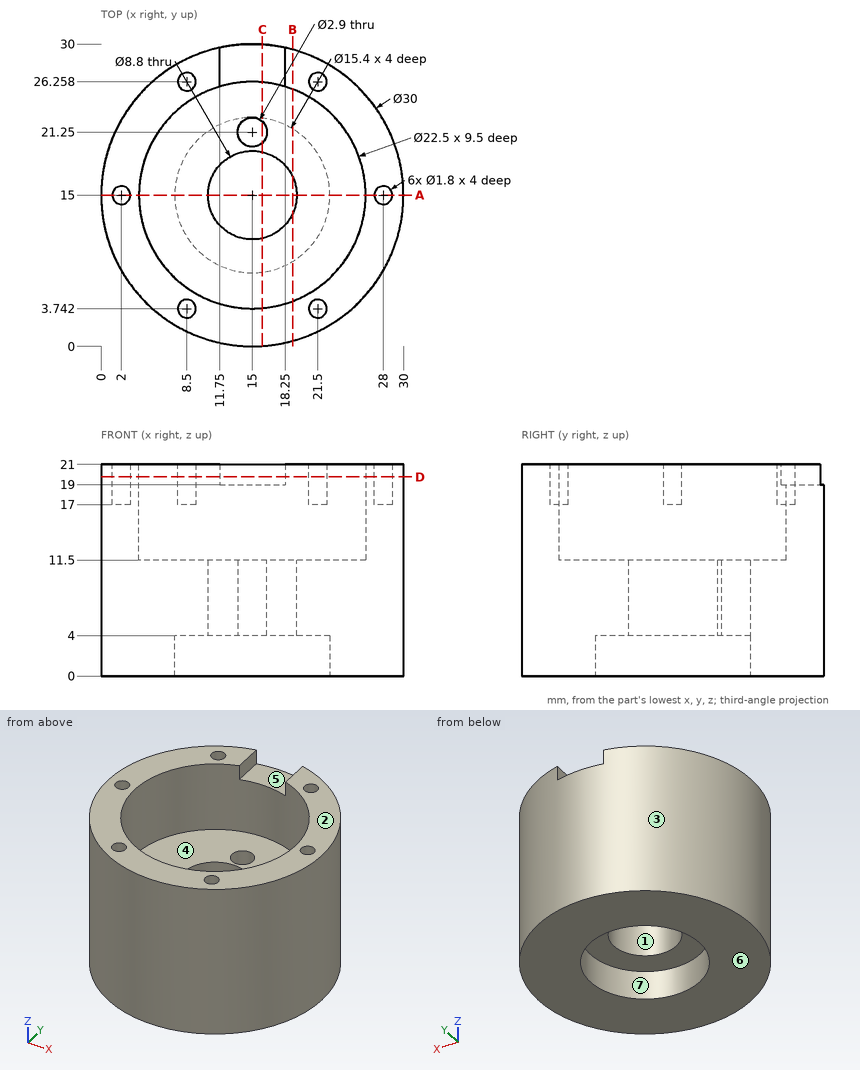
The drawing under review shows one solid part. Ordinate dimensions are in mm from its lowest x, y, z. A direction names the side the tool comes from. Give positions to 0.01 mm unless a question says otherwise; leave off trailing zeros. Order: outer loops, then holes, each group sorted by start corner. A loop starts at its lowest first (then second) coordinate and runs counter-clockwise, first axis right, second up. Notation, with made-up numbers: M 37.25,61.5 L 66.25,61.5 A24 ccw 66.25,76.5 Z; hole C 50,62.25 d6. An arc over 180 degrees is marked long. One line per question, with ' | ' between items. Start each with the question number.
Q1. Machinability: for the marked faces 4, 5, 6 and 7, which of the approach directions +Z, -Z, +X, -X, +Y, -Y give a long, thin tool a straight path to every point of the face, cutting with its end or side? Answer none if there is none.
Q2. We need section C-C (x = 16). State how many separate pieces and enclosed holes the cut face has, plus the area to 3 significant figures.
Q3. We need section A-A (y = 15). Write out the cut boundary in (x, z).
Q4. The part is to be moulded in two halves that separate along Y. For the marked faces 1, 2 and 3, say which applies: +Y half, -Y half, draft (parallel to the pull), parting line (faces both ways), or undercut.
Q5. We need section D-D (z = 19.75). Write out the cut boundary in (x, y), plus the area to 3 significant figures.
Q6. We need section B-B (x = 19). Write out the cut boundary in (y, z) (1 decimal).
Q7. For L1, parallel to X at y = 15, z = 3; L2, parallel to Y at x = 21.5, z = 18.3; L3, parallel to Y at x = 15, z = 8.5, list the stretches that pass through material, from the lowest coordinate up. Write a range as [from, to].
Q8. For pin 1 Ø5.5 at (x, y) = (15, 15) entering from +Z; pin 2 Ø2 at (y, z) = (28, 20.5) entering from +X; pin 3 Ø12 at (x, z) = (23.5, 15) entering from +Y; pin 4 Ø0.9 at (x, y) = (8.5, 4) entering from +Z, all flat-tipped, find the tip position at first contact; note any pin that passes through.
Returned:
1) face 4: +Z | face 5: +Z, +Y | face 6: -Z, +X, -X, +Y, -Y | face 7: -Z
2) separate pieces: 3 | enclosed holes: 0 | area: 267 mm2
3) outline: M 0,0 L 7.3,0 L 7.3,4 L 10.6,4 L 10.6,11.5 L 3.75,11.5 L 3.75,21 L 2.9,21 L 2.9,17 L 1.1,17 L 1.1,21 L 0,21 Z; M 19.4,4 L 22.7,4 L 22.7,0 L 30,0 L 30,21 L 28.9,21 L 28.9,17 L 27.1,17 L 27.1,21 L 26.25,21 L 26.25,11.5 L 19.4,11.5 Z
4) face 1: undercut | face 2: draft | face 3: parting line
5) outline: M 11.75,25.77 L 11.75,29.64 A15 ccw long 18.25,29.64 L 18.25,25.77 A11.25 cw long Z; hole C 2,15 d1.8; hole C 8.5,3.74 d1.8; hole C 8.5,26.26 d1.8; hole C 21.5,3.74 d1.8; hole C 21.5,26.26 d1.8; hole C 28,15 d1.8 | area: 269 mm2
6) outline: M 0.5,0 L 8.4,0 L 8.4,4 L 13.2,4 L 13.2,11.5 L 4.5,11.5 L 4.5,21 L 0.5,21 Z; M 16.8,4 L 21.6,4 L 21.6,0 L 29.5,0 L 29.5,21 L 25.5,21 L 25.5,11.5 L 16.8,11.5 Z
7) L1: [0, 7.3], [22.7, 30] | L2: [1.48, 2.84], [4.64, 5.82], [24.18, 25.36], [27.16, 28.52] | L3: [0, 10.6], [19.4, 19.8], [22.7, 30]
8) pin 1: through | pin 2: x = 24 | pin 3: y = 29.79 | pin 4: z = 17
